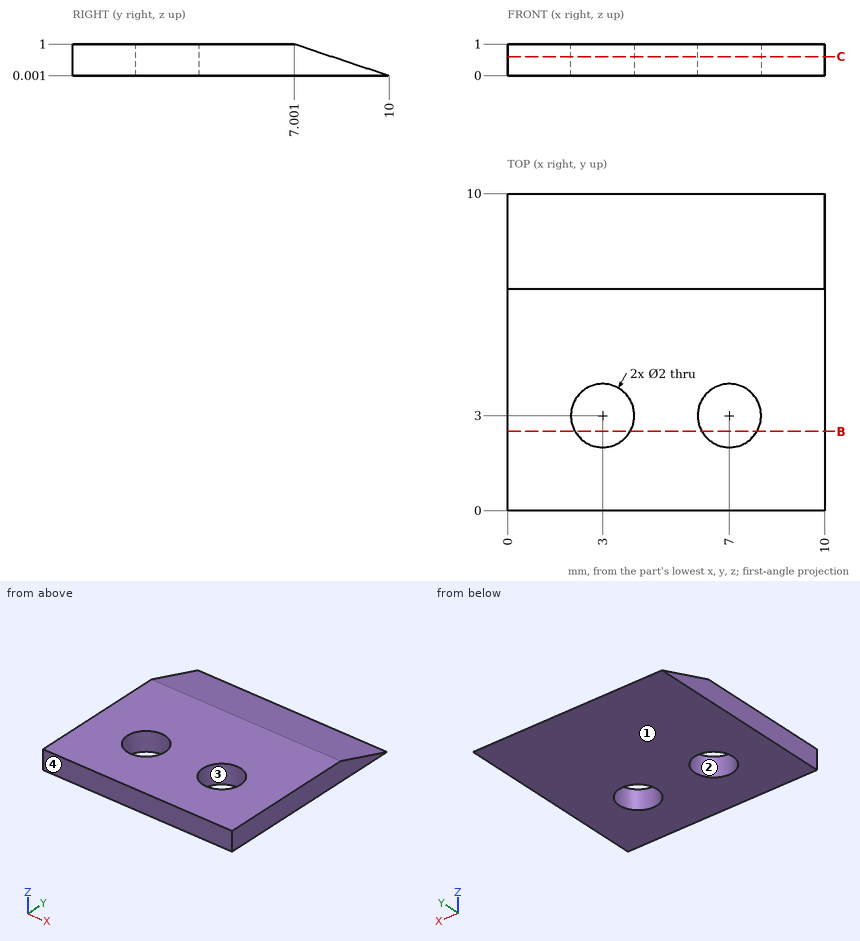
Verification items for this drawing (mm, ordinates from the low corner). Coordinates: 2 decimals unless noted, no trailing zeros. Loops run counter-clockwise (first coordinate to the right, second up) from the corner with the lowest first, then second, coordinate; pieces in that order, holes last. Notation, with made-up numbers: (-34, -26) -> (-15, -26) arc R33 ccw to (-15, 5) -> close; hole circle Ø9 at (-26, -26). An arc over 180 degrees is marked (long way). Put each result on its own line as item: value.
1. Section check C-C, the plane z = 0.6. Record the boundary of the cut face in (x, y).
Result set:
outline: (0, 0) -> (10, 0) -> (10, 8.2) -> (0, 8.2) -> close; hole circle Ø2 at (3, 3); hole circle Ø2 at (7, 3)
2. Gauge pin test, flat end, axial feed: P1, Ø1.6, axis at x = 7, y = 3, coming from the +Z side. Record the tip position at first contact, or that the pin passes through.
Result set:
P1: passes through
3. Section check B-B, the plane y = 2.5. Record the boundary of the cut face in (x, z).
Result set:
outline: (0, 0) -> (2.13, 0) -> (2.13, 1) -> (0, 1) -> close; (3.87, 0) -> (6.13, 0) -> (6.13, 1) -> (3.87, 1) -> close; (7.87, 0) -> (10, 0) -> (10, 1) -> (7.87, 1) -> close
4. Mould release check, pull along Y, two halves, no side actions. Record for the marked faces 1, 2, 3 and 4: pulls with the +Y half, pulls with the -Y half, needs draft (parallel to the pull), parting line crosses it, or undercut.
Result set:
face 1: needs draft
face 2: undercut
face 3: undercut
face 4: pulls with the -Y half
5. Thickness scan on line 1 (X direction, y = 3.5, z = 0.35) (1 decimal); line 2 (Z direction, x = 1.25, y = 7.5) (1 decimal); line 3 (Z direction, x = 9.25, y = 7.25). Record the ranges inside material, lowest first.
Result set:
line 1: x = 0 to 2.1, 3.9 to 6.1, 7.9 to 10
line 2: z = 0 to 0.8
line 3: z = 0 to 0.92
